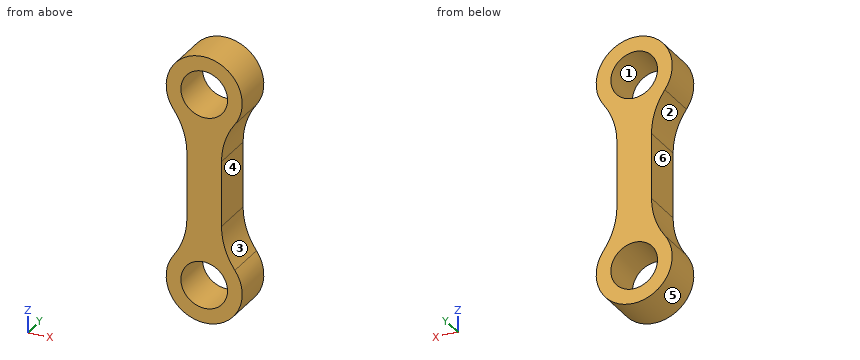
```python
from build123d import *

# Parameters (mm, degrees)
F0_R     = 1.6875
F1_DEPTH = 3
F2_R     = 5


with BuildPart() as f1:
    # F0 (on Front) → F1 (new body)
    with BuildSketch(Plane.XZ):
        with BuildLine():
            Line((-1.25, 11.433086), (-1.25, 2.44949))
            ThreePointArc((-1.25, 2.44949), (0, -2.75), (1.25, 2.44949))
            Line((1.25, 2.44949), (1.25, 11.433086))
            ThreePointArc((1.25, 11.433086), (0, 16.632576), (-1.25, 11.433086))
        make_face()
        Circle(F0_R, mode=Mode.SUBTRACT)
        with Locations((0, 13.882576)):
            Circle(F0_R, mode=Mode.SUBTRACT)
    extrude(amount=F1_DEPTH)

    # F2
    f2_edges = [f1.edges().sort_by_distance(p)[0] for p in [
        (1.25, -1.5, 2.44949),
        (-1.25, -1.5, 2.44949),
        (-1.25, -1.5, 11.433086),
        (1.25, -1.5, 11.433086),
    ]]
    fillet(f2_edges, radius=F2_R)


solid = f1.part
```
CAD build for the part. Positions are in the model's coordinates, mm. Face numbers are marked on the shaded views. A direction names the side the tool comes from. Coordinates: 2 decimals unless noted, no trailing zeros. Order: outer loops, then holes, each group sorted by start corner. A loop starts at its lowest first (then second) coordinate and runs counter-clockwise, first axis right, second up. Notation, with made-up numbers: (62, 11.5) - (108, 11.5) arc R9 ccw to (108, 21.5) - close; hole circle Ø8 at (77, 18.25). An arc over 180 degrees is marked (long way). Use a Markdown table: item, result. Add a question column.
(1) Which spindle directions (+Z, -Z, +X, -X, +Y, -Y) get a long thin tool onto all of the face, cutting with end or side? Do the marked faces 4, 5 and 6. Say none if no direction does.
(2) Drill centre lines: line 1 along Z through (x, y) = (0, -2.1); line 2 along Z through (x, y) = (-0.3, -2.45); line 3 along X through (y, z) = (-1.55, -0.25). Where is each one in solid material? Low to high. Write a range as [from, to].
(3) Pull direction X, two halves, no side cores. Call the marked faces 1, 2 and 3: +X half, -X half, draft (parallel to the pull), parting line (faces both ways), or undercut.
(4) Saw through at A-A (z = 0). Give the cut face in (x, y), then the cut area to 4 significant figures.
(5) Flat gauge pin, fed straight in: pin 1 (0.9 mm diameter, centred on y = -2, z = 7, fed in from -X). Where does the tip first touch, or does it go through?
(6) Saw through at C-C (y = -0.95). Count the separate pieces of the cut face and the enclosed holes in it, then the cut area to 3 significant figures.
(7) Saw through at D-D (z = 5.25). Give the cut face in (x, y), then the cut area to 3 significant figures.
(8) Saw through at B-B (x = 0). Give the cut face in (y, z).
Solved:
| question | item | result |
|---|---|---|
| 1 | face 4 | +X, +Y, -Y |
| 1 | face 5 | +Y, -Y |
| 1 | face 6 | -X, +Y, -Y |
| 2 | line 1 | z = [-2.75, -1.69], [1.69, 12.2], [15.57, 16.63] |
| 2 | line 2 | z = [-2.73, -1.66], [1.66, 12.22], [15.54, 16.62] |
| 2 | line 3 | x = [-2.74, -1.67], [1.67, 2.74] |
| 3 | face 1 | undercut |
| 3 | face 2 | -X half |
| 3 | face 3 | +X half |
| 4 | outline | (-2.75, -3) - (-1.69, -3) - (-1.69, 0) - (-2.75, 0) - close; (1.69, -3) - (2.75, -3) - (2.75, 0) - (1.69, 0) - close |
| 4 | area | 6.375 mm² |
| 5 | pin 1 | stops at x = -1.25 |
| 6 | separate pieces | 1 |
| 6 | enclosed holes | 2 |
| 6 | area | 52.9 mm² |
| 7 | outline | (-1.25, -3) - (1.25, -3) - (1.25, 0) - (-1.25, 0) - close |
| 7 | area | 7.50 mm² |
| 8 | outline | (-3, -2.75) - (0, -2.75) - (0, -1.69) - (-3, -1.69) - close; (-3, 1.69) - (0, 1.69) - (0, 12.2) - (-3, 12.2) - close; (-3, 15.57) - (0, 15.57) - (0, 16.63) - (-3, 16.63) - close |
